```python
from build123d import *

# Parameters (mm, degrees)
SKETCH1_W           = 355.6
SKETCH1_H           = 139.7
BOSS_EXTRUDE1_DEPTH = 5.08
SKETCH2_R           = 16.7005
CUT_EXTRUDE1_DEPTH  = 6.08
SKETCH4_W           = 5.08
SKETCH4_H           = 9.525
SKETCH4_W_2         = 9.525
SKETCH4_H_2         = 5.08
CUT_EXTRUDE3_DEPTH  = 6.08


with BuildPart() as part:
    # Sketch1 → Boss-Extrude1 (new body)
    with BuildSketch(Plane(origin=(0, 0, 0), x_dir=(1, 0, 0), z_dir=(0, 1, 0))):
        Rectangle(SKETCH1_W, SKETCH1_H)
    extrude(amount=BOSS_EXTRUDE1_DEPTH)

    # Sketch2 → Cut-Extrude1 (cut, through all)
    with BuildSketch(Plane(origin=(0, 5.08, 0), x_dir=(1, 0, 0), z_dir=(0, 1, 0))):
        with Locations((-79.375, -12.7)):
            Circle(SKETCH2_R)
        with Locations((79.375, -12.7)):
            Circle(SKETCH2_R)
    extrude(amount=-CUT_EXTRUDE1_DEPTH, mode=Mode.SUBTRACT)

    # Sketch4 → Cut-Extrude3 (cut, through all)
    with BuildSketch(Plane(origin=(0, 5.08, 0), x_dir=(1, 0, 0), z_dir=(0, 1, 0))):
        with Locations((-22.5044, -7.9629)):
            Rectangle(SKETCH4_W, SKETCH4_H)
        with Locations((-20.2819, -32.4104)):
            Rectangle(SKETCH4_W_2, SKETCH4_H_2)
        with Locations((9.8806, -32.4104)):
            Rectangle(SKETCH4_W_2, SKETCH4_H_2)
        with Locations((40.0431, -32.4104)):
            Rectangle(SKETCH4_W_2, SKETCH4_H_2)
        with Locations((42.2656, -7.9629)):
            Rectangle(SKETCH4_W, SKETCH4_H)
    extrude(amount=-CUT_EXTRUDE3_DEPTH, mode=Mode.SUBTRACT)


solid = part.part
```
The model under review builds one solid part; all positions refer to its coordinate system, in mm. Give positions to 0.01 mm unless a question says otherwise; leave off trailing zeros. Order: outer loops, then holes, each group sorted by start corner. A loop starts at its lowest first (then second) coordinate and runs counter-clockwise, first axis right, second up. Notation, with made-up numbers: (85.25, 52) - (100.25, 52) arc R20 cw to (100.25, 68) - close; hole circle Ø2 at (-13.75, 13.5). An arc over 180 degrees is marked (long way). Use CSV: the item, a comma, the result in double quotes. Start each with the question number.
Q1. We need section B-B, the plane z = 26. Write out the cut boundary in (x, y), and give its area (3 significant figures).
Q2. We need section C-C, the plane x = 85.5. Write out the cut boundary in (y, z), and give its area (3 significant figures).
Q3. We need section A-A, the plane y = 2.75. State how many separate pieces and enclosed holes the cut face has, and give its area (3 significant figures).
Q4. To check wall thickness, follow line 1 along X through (y, z) = (0.4, 20.5); line 2 along Z through (x, y) = (-16, 3.95); line 3 along X through (y, z) = (0.6, 22.5). State the ranges of each line that lie inside material, in increasing order. Write a range as [from, to].
Q5. The part is to be moulded in two halves that separate along Z. For faces 1 (the flat face through (-2, 0, -1)), 2 (the cylindrical face through (-63.446, 2.576, 7.684)), 3 (the cylindrical face through (95.304, 2.576, 7.684)), say which applies: +Z half, -Z half, draft (parallel to the pull), parting line (faces both ways), or undercut.
Outcome:
1,outline,"(-177.8, 0) - (-89.48, 0) - (-89.48, 5.08) - (-177.8, 5.08) - close; (-69.27, 0) - (69.27, 0) - (69.27, 5.08) - (-69.27, 5.08) - close; (89.48, 0) - (177.8, 0) - (177.8, 5.08) - (89.48, 5.08) - close"
1,area,"1,600 mm^2"
2,outline,"(0, -69.85) - (5.08, -69.85) - (5.08, -2.84) - (0, -2.84) - close; (0, 28.24) - (5.08, 28.24) - (5.08, 69.85) - (0, 69.85) - close"
2,area,"552 mm^2"
3,separate pieces,"1"
3,enclosed holes,"7"
3,area,"47,700 mm^2"
4,line 1,"x = [-177.8, -94.14], [-64.61, 64.61], [94.14, 177.8]"
4,line 2,"z = [-69.85, 29.87], [34.95, 69.85]"
4,line 3,"x = [-177.8, -92.9], [-65.85, 65.85], [92.9, 177.8]"
5,face 1,"draft"
5,face 2,"undercut"
5,face 3,"undercut"
